Here's how the part is built. I have some questions about the finished solid (model axes, mm). Face numbers are marked on the shaded views. A direction names the side the tool comes from. Give positions to 0.01 mm unless a question says otherwise; leave off trailing zeros. Write each loop counter-clockwise with the first axis right and the second up, starting at its lowest first coordinate (ties: lowest second). Pieces come first, ordered by that corner, then holes. Notation, with made-up numbers: (34, 54.5) - (58, 54.5) arc R9 cw to (58, 61.5) - close; hole circle Ø5 at (20.25, 85). An arc over 180 degrees is marked (long way). Write each question's results on one line, items separated by ' | '. Start each with the question number.
Item 1: Suppose I cut it at B-B on x = 39.5. List the corners of the cut face in (y, z) for me.
Item 2: Suppose I cut it at A-A on y = 0. List the corners of the cut face in (x, z) for me, then the cut area to 4 significant figures.
Item 3: We'd pull the mould along X, two halves only. Please class the marked faces 4, 5 and 6: +X half, -X half, draft (parallel to the pull), parting line (faces both ways), or undercut.
Item 4: Which directions (+Z, -Z, +X, -X, +Y, -Y) give clear straight access to the entire face, cutting with the end or side of a thin tool? Please do the marked faces 1, 2 and 3.
Item 5: Please list where these lines run through material, in increasing order: line 1 along X through (y, z) = (17, 4); line 2 along Z through (x, y) = (43.5, -10); line 3 along X through (y, z) = (-20, 2.5).
Item 6: Suppose I cut it at D-D on z = -22. List the corners of the cut face in (x, y) for me.
Item 7: Will these pins go through, and if not, where does the flat tip stop? P1, Ø9.5, axis at x = 0, y = 35, coming from the -Z side; P2, Ø12, axis at x = -1.5, z = -7.5, coming from the -Y side; P3, Ø3, axis at x = 2.5, z = -31.5, coming from the +Y side; P4, Ø9, axis at x = 7, y = -1.5, coming from the -Z side.
Item 8: Suppose I cut it at C-C on y = -33. List the corners of the cut face in (x, z) for me, then the cut area to 3 significant figures.
```python
from build123d import *

# Parameters (mm, degrees)
SKETCH1_R           = 50
BOSS_EXTRUDE1_DEPTH = 15
SKETCH2_R           = 25
BOSS_EXTRUDE2_DEPTH = 70
BOSS_EXTRUDE3_DEPTH = 15
SKETCH5_R           = 15
CUT_EXTRUDE1_DEPTH  = 85
SKETCH6_R           = 5
CUT_EXTRUDE2_DEPTH  = 30
SKETCH7_R           = 6
CUT_EXTRUDE3_DEPTH  = 30


with BuildPart() as part:
    # Sketch1 → Boss-Extrude1 (new body)
    with BuildSketch(Plane.XY):
        Circle(SKETCH1_R)
    extrude(amount=BOSS_EXTRUDE1_DEPTH)

    # Sketch2 → Boss-Extrude2 (add)
    with BuildSketch(Plane(origin=(0, 0, 0), x_dir=(-1, 0, 0), z_dir=(0, 0, -1))):
        Circle(SKETCH2_R)
    extrude(amount=BOSS_EXTRUDE2_DEPTH)

    # Sketch4 → Boss-Extrude3 (add)
    with BuildSketch(Plane(origin=(0, 0, -70), x_dir=(-1, 0, 0), z_dir=(0, 0, -1))):
        with BuildLine():
            Line((-50, 12.5), (-6.462424595, 24.15030162))
            ThreePointArc((-6.462424595, 24.15030162), (0, 25), (6.462424595, 24.15030162))
            Line((6.462424595, 24.15030162), (50, 12.5))
            ThreePointArc((50, 12.5), (62.5, 0), (50, -12.5))
            Line((50, -12.5), (6.462424595, -24.15030162))
            ThreePointArc((6.462424595, -24.15030162), (0, -25), (-6.462424595, -24.15030162))
            Line((-6.462424595, -24.15030162), (-50, -12.5))
            ThreePointArc((-50, -12.5), (-62.5, 0), (-50, 12.5))
        make_face()
    extrude(amount=BOSS_EXTRUDE3_DEPTH)

    # Sketch5 → Cut-Extrude1 (cut)
    with BuildSketch(Plane(origin=(0, 0, -85), x_dir=(-1, 0, 0), z_dir=(0, 0, -1))):
        Circle(SKETCH5_R)
    extrude(amount=-CUT_EXTRUDE1_DEPTH, mode=Mode.SUBTRACT)

    # Sketch6 → Cut-Extrude2 (cut)
    with BuildSketch(Plane(origin=(0, 0, -85), x_dir=(-1, 0, 0), z_dir=(0, 0, -1))):
        with Locations((50, 0)):
            Circle(SKETCH6_R)
        with Locations((-50, 0)):
            Circle(SKETCH6_R)
    extrude(amount=-CUT_EXTRUDE2_DEPTH, mode=Mode.SUBTRACT)

    # Sketch7 → Cut-Extrude3 (cut)
    with BuildSketch(Plane(origin=(0, 0, 0), x_dir=(-1, 0, 0), z_dir=(0, 0, -1))):
        with Locations((0, 35)):
            Circle(SKETCH7_R)
        with Locations((30.310889132, 17.5)):
            Circle(SKETCH7_R)
        with Locations((30.310889132, -17.5)):
            Circle(SKETCH7_R)
        with Locations((0, -35)):
            Circle(SKETCH7_R)
        with Locations((-30.310889132, -17.5)):
            Circle(SKETCH7_R)
        with Locations((-30.310889132, 17.5)):
            Circle(SKETCH7_R)
    extrude(amount=-CUT_EXTRUDE3_DEPTH, mode=Mode.SUBTRACT)


solid = part.part
```
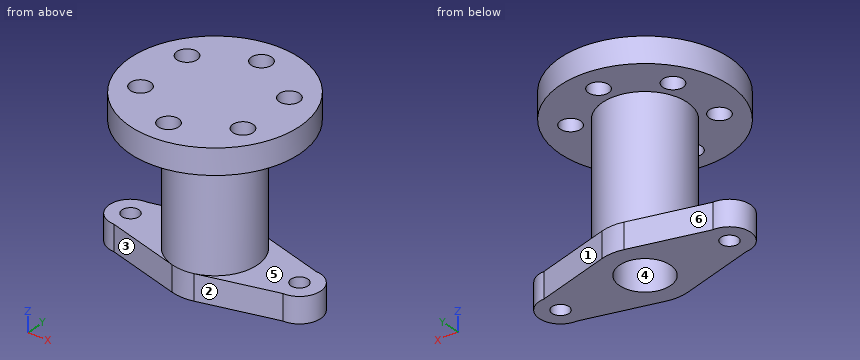
Checked values:
1) outline: (-30.66, 0) - (30.66, 0) - (30.66, 15) - (-30.66, 15) - close; (-15.31, -85) - (15.31, -85) - (15.31, -70) - (-15.31, -70) - close
2) outline: (-62.5, -85) - (-55, -85) - (-55, -70) - (-62.5, -70) - close; (-50, 0) - (-25, 0) - (-25, -70) - (-45, -70) - (-45, -85) - (-15, -85) - (-15, 0) - (15, 0) - (15, -85) - (45, -85) - (45, -70) - (25, -70) - (25, 0) - (50, 0) - (50, 15) - (-50, 15) - close; (55, -85) - (62.5, -85) - (62.5, -70) - (55, -70) - close | area: 4,025 mm^2
3) face 4: undercut | face 5: draft | face 6: -X half
4) face 1: -Z, +X, +Y | face 2: -Z, +X, -Y | face 3: -Z, -X, -Y
5) line 1: x = -47.02 to -36.29, -24.33 to 24.33, 36.29 to 47.02 | line 2: z = -85 to -70, 0 to 15 | line 3: x = -45.83 to -35.77, -24.86 to 24.86, 35.77 to 45.83
6) outline: circle Ø50 at (0, 0); hole circle Ø30 at (0, 0)
7) P1: passes through | P2: stops at y = -25 | P3: stops at y = 24.98 | P4: stops at z = 0
8) outline: (-37.56, 0) - (-5.66, 0) - (-5.66, 15) - (-37.56, 15) - close; (5.66, 0) - (37.56, 0) - (37.56, 15) - (5.66, 15) - close | area: 957 mm^2
